from build123d import *

# Parameters (mm, degrees)
BOSS_EXTRUDE1_DEPTH       = 360
CUT_EXTRUDE1_REACH        = 4
SKETCH2_R                 = 2.25
SKETCH3_R                 = 2.25
CUT_EXTRUDE2_DEPTH        = 2
LPATTERN1_COUNT           = 5
LPATTERN1_PITCH           = 25.65625
LPATTERN2_COUNT           = 3
LPATTERN2_PITCH           = 124.1875
LPATTERN2_COPY_1_SKETCH_R = 2.25
LPATTERN2_COPY_1_DEPTH    = 2
LPATTERN2_COPY_2_SKETCH_R = 2.25
LPATTERN2_COPY_2_DEPTH    = 2
LPATTERN2_COPY_3_SKETCH_R = 2.25
LPATTERN2_COPY_3_DEPTH    = 2
LPATTERN2_COPY_4_SKETCH_R = 2.25
LPATTERN2_COPY_4_DEPTH    = 2
LPATTERN2_COPY_5_SKETCH_R = 2.25
LPATTERN2_COPY_5_DEPTH    = 2
LPATTERN2_COPY_6_SKETCH_R = 2.25
LPATTERN2_COPY_6_DEPTH    = 2
LPATTERN2_COPY_7_SKETCH_R = 2.25
LPATTERN2_COPY_7_DEPTH    = 2
LPATTERN2_COPY_8_SKETCH_R = 2.25
LPATTERN2_COPY_8_DEPTH    = 2


with BuildPart() as part:
    # Sketch1 → Boss-Extrude1 (new body)
    with BuildSketch(Plane(origin=(0, 0, 0), x_dir=(1, 0, 0), z_dir=(0, 1, 0))):
        Polygon((0, 0), (15, 0), (15, 12), (13, 12), (13, 2), (0, 2), align=None)
    extrude(amount=BOSS_EXTRUDE1_DEPTH)

    # Sketch2 → Cut-Extrude1 (cut, up to next)
    with BuildSketch(Plane.ZY.offset(-13), mode=Mode.PRIVATE) as cut_extrude1_sk1:
        with Locations((-4.5, 329.8125)):
            Circle(SKETCH2_R)
    cut_extrude1_tool1 = extrude(cut_extrude1_sk1.sketch, amount=-CUT_EXTRUDE1_REACH, mode=Mode.PRIVATE) & part.part
    add(cut_extrude1_tool1.solids().sort_by_distance((13, 329.8125, -4.5))[0], mode=Mode.SUBTRACT)
    # Sketch2 → Cut-Extrude1 (cut, up to next)
    with BuildSketch(Plane.ZY.offset(-13), mode=Mode.PRIVATE) as cut_extrude1_sk2:
        with Locations((-4.5, 304.125)):
            Circle(SKETCH2_R)
    cut_extrude1_tool2 = extrude(cut_extrude1_sk2.sketch, amount=-CUT_EXTRUDE1_REACH, mode=Mode.PRIVATE) & part.part
    add(cut_extrude1_tool2.solids().sort_by_distance((13, 304.125, -4.5))[0], mode=Mode.SUBTRACT)
    # Sketch2 → Cut-Extrude1 (cut, up to next)
    with BuildSketch(Plane.ZY.offset(-13), mode=Mode.PRIVATE) as cut_extrude1_sk3:
        with Locations((-4.5, 278.4375)):
            Circle(SKETCH2_R)
    cut_extrude1_tool3 = extrude(cut_extrude1_sk3.sketch, amount=-CUT_EXTRUDE1_REACH, mode=Mode.PRIVATE) & part.part
    add(cut_extrude1_tool3.solids().sort_by_distance((13, 278.4375, -4.5))[0], mode=Mode.SUBTRACT)
    # Sketch2 → Cut-Extrude1 (cut, up to next)
    with BuildSketch(Plane.ZY.offset(-13), mode=Mode.PRIVATE) as cut_extrude1_sk4:
        with Locations((-4.5, 252.75)):
            Circle(SKETCH2_R)
    cut_extrude1_tool4 = extrude(cut_extrude1_sk4.sketch, amount=-CUT_EXTRUDE1_REACH, mode=Mode.PRIVATE) & part.part
    add(cut_extrude1_tool4.solids().sort_by_distance((13, 252.75, -4.5))[0], mode=Mode.SUBTRACT)
    # Sketch2 → Cut-Extrude1 (cut, up to next)
    with BuildSketch(Plane.ZY.offset(-13), mode=Mode.PRIVATE) as cut_extrude1_sk5:
        with Locations((-4.5, 231.375)):
            Circle(SKETCH2_R)
    cut_extrude1_tool5 = extrude(cut_extrude1_sk5.sketch, amount=-CUT_EXTRUDE1_REACH, mode=Mode.PRIVATE) & part.part
    add(cut_extrude1_tool5.solids().sort_by_distance((13, 231.375, -4.5))[0], mode=Mode.SUBTRACT)
    # Sketch2 → Cut-Extrude1 (cut, up to next)
    with BuildSketch(Plane.ZY.offset(-13), mode=Mode.PRIVATE) as cut_extrude1_sk6:
        with Locations((-4.5, 205.6875)):
            Circle(SKETCH2_R)
    cut_extrude1_tool6 = extrude(cut_extrude1_sk6.sketch, amount=-CUT_EXTRUDE1_REACH, mode=Mode.PRIVATE) & part.part
    add(cut_extrude1_tool6.solids().sort_by_distance((13, 205.6875, -4.5))[0], mode=Mode.SUBTRACT)
    # Sketch2 → Cut-Extrude1 (cut, up to next)
    with BuildSketch(Plane.ZY.offset(-13), mode=Mode.PRIVATE) as cut_extrude1_sk7:
        with Locations((-4.5, 180)):
            Circle(SKETCH2_R)
    cut_extrude1_tool7 = extrude(cut_extrude1_sk7.sketch, amount=-CUT_EXTRUDE1_REACH, mode=Mode.PRIVATE) & part.part
    add(cut_extrude1_tool7.solids().sort_by_distance((13, 180, -4.5))[0], mode=Mode.SUBTRACT)
    # Sketch2 → Cut-Extrude1 (cut, up to next)
    with BuildSketch(Plane.ZY.offset(-13), mode=Mode.PRIVATE) as cut_extrude1_sk8:
        with Locations((-4.5, 154.3125)):
            Circle(SKETCH2_R)
    cut_extrude1_tool8 = extrude(cut_extrude1_sk8.sketch, amount=-CUT_EXTRUDE1_REACH, mode=Mode.PRIVATE) & part.part
    add(cut_extrude1_tool8.solids().sort_by_distance((13, 154.3125, -4.5))[0], mode=Mode.SUBTRACT)
    # Sketch2 → Cut-Extrude1 (cut, up to next)
    with BuildSketch(Plane.ZY.offset(-13), mode=Mode.PRIVATE) as cut_extrude1_sk9:
        with Locations((-4.5, 128.625)):
            Circle(SKETCH2_R)
    cut_extrude1_tool9 = extrude(cut_extrude1_sk9.sketch, amount=-CUT_EXTRUDE1_REACH, mode=Mode.PRIVATE) & part.part
    add(cut_extrude1_tool9.solids().sort_by_distance((13, 128.625, -4.5))[0], mode=Mode.SUBTRACT)
    # Sketch2 → Cut-Extrude1 (cut, up to next)
    with BuildSketch(Plane.ZY.offset(-13), mode=Mode.PRIVATE) as cut_extrude1_sk10:
        with Locations((-4.5, 107.25)):
            Circle(SKETCH2_R)
    cut_extrude1_tool10 = extrude(cut_extrude1_sk10.sketch, amount=-CUT_EXTRUDE1_REACH, mode=Mode.PRIVATE) & part.part
    add(cut_extrude1_tool10.solids().sort_by_distance((13, 107.25, -4.5))[0], mode=Mode.SUBTRACT)
    # Sketch2 → Cut-Extrude1 (cut, up to next)
    with BuildSketch(Plane.ZY.offset(-13), mode=Mode.PRIVATE) as cut_extrude1_sk11:
        with Locations((-4.5, 81.5625)):
            Circle(SKETCH2_R)
    cut_extrude1_tool11 = extrude(cut_extrude1_sk11.sketch, amount=-CUT_EXTRUDE1_REACH, mode=Mode.PRIVATE) & part.part
    add(cut_extrude1_tool11.solids().sort_by_distance((13, 81.5625, -4.5))[0], mode=Mode.SUBTRACT)
    # Sketch2 → Cut-Extrude1 (cut, up to next)
    with BuildSketch(Plane.ZY.offset(-13), mode=Mode.PRIVATE) as cut_extrude1_sk12:
        with Locations((-4.5, 55.875)):
            Circle(SKETCH2_R)
    cut_extrude1_tool12 = extrude(cut_extrude1_sk12.sketch, amount=-CUT_EXTRUDE1_REACH, mode=Mode.PRIVATE) & part.part
    add(cut_extrude1_tool12.solids().sort_by_distance((13, 55.875, -4.5))[0], mode=Mode.SUBTRACT)
    # Sketch2 → Cut-Extrude1 (cut, up to next)
    with BuildSketch(Plane.ZY.offset(-13), mode=Mode.PRIVATE) as cut_extrude1_sk13:
        with Locations((-4.5, 30.1875)):
            Circle(SKETCH2_R)
    cut_extrude1_tool13 = extrude(cut_extrude1_sk13.sketch, amount=-CUT_EXTRUDE1_REACH, mode=Mode.PRIVATE) & part.part
    add(cut_extrude1_tool13.solids().sort_by_distance((13, 30.1875, -4.5))[0], mode=Mode.SUBTRACT)
    # Sketch2 → Cut-Extrude1 (cut, up to next)
    with BuildSketch(Plane.ZY.offset(-13), mode=Mode.PRIVATE) as cut_extrude1_sk14:
        with Locations((-4.5, 4.5)):
            Circle(SKETCH2_R)
    cut_extrude1_tool14 = extrude(cut_extrude1_sk14.sketch, amount=-CUT_EXTRUDE1_REACH, mode=Mode.PRIVATE) & part.part
    add(cut_extrude1_tool14.solids().sort_by_distance((13, 4.5, -4.5))[0], mode=Mode.SUBTRACT)
    # Sketch2 → Cut-Extrude1 (cut, up to next)
    with BuildSketch(Plane.ZY.offset(-13), mode=Mode.PRIVATE) as cut_extrude1_sk15:
        with Locations((-4.5, 355.5)):
            Circle(SKETCH2_R)
    cut_extrude1_tool15 = extrude(cut_extrude1_sk15.sketch, amount=-CUT_EXTRUDE1_REACH, mode=Mode.PRIVATE) & part.part
    add(cut_extrude1_tool15.solids().sort_by_distance((13, 355.5, -4.5))[0], mode=Mode.SUBTRACT)

    # Sketch3 → Cut-Extrude2 (cut)
    with BuildSketch(Plane.XY):
        with Locations((7.5, 355.5)):
            Circle(SKETCH3_R)
    cut_extrude2 = extrude(amount=-CUT_EXTRUDE2_DEPTH, mode=Mode.SUBTRACT)

    # LPattern1: Cut-Extrude2 ×5
    with Locations(*[(0, -i * LPATTERN1_PITCH, 0) for i in range(1, LPATTERN1_COUNT)]):
        add(cut_extrude2, mode=Mode.SUBTRACT)

    # LPattern2: Cut-Extrude2 ×3
    with Locations(*[(0, -i * LPATTERN2_PITCH, 0) for i in range(1, LPATTERN2_COUNT)]):
        add(cut_extrude2, mode=Mode.SUBTRACT)

    # LPattern2 copy 1 sketch → LPattern2 copy 1 (cut)
    with BuildSketch(Plane(origin=(0, -149.84375, 0), x_dir=(1, 0, 0), z_dir=(0, 0, 1))):
        with Locations((7.5, 355.5)):
            Circle(LPATTERN2_COPY_1_SKETCH_R)
    extrude(amount=-LPATTERN2_COPY_1_DEPTH, mode=Mode.SUBTRACT)

    # LPattern2 copy 2 sketch → LPattern2 copy 2 (cut)
    with BuildSketch(Plane(origin=(0, -274.03125, 0), x_dir=(1, 0, 0), z_dir=(0, 0, 1))):
        with Locations((7.5, 355.5)):
            Circle(LPATTERN2_COPY_2_SKETCH_R)
    extrude(amount=-LPATTERN2_COPY_2_DEPTH, mode=Mode.SUBTRACT)

    # LPattern2 copy 3 sketch → LPattern2 copy 3 (cut)
    with BuildSketch(Plane(origin=(0, -175.5, 0), x_dir=(1, 0, 0), z_dir=(0, 0, 1))):
        with Locations((7.5, 355.5)):
            Circle(LPATTERN2_COPY_3_SKETCH_R)
    extrude(amount=-LPATTERN2_COPY_3_DEPTH, mode=Mode.SUBTRACT)

    # LPattern2 copy 4 sketch → LPattern2 copy 4 (cut)
    with BuildSketch(Plane(origin=(0, -299.6875, 0), x_dir=(1, 0, 0), z_dir=(0, 0, 1))):
        with Locations((7.5, 355.5)):
            Circle(LPATTERN2_COPY_4_SKETCH_R)
    extrude(amount=-LPATTERN2_COPY_4_DEPTH, mode=Mode.SUBTRACT)

    # LPattern2 copy 5 sketch → LPattern2 copy 5 (cut)
    with BuildSketch(Plane(origin=(0, -201.15625, 0), x_dir=(1, 0, 0), z_dir=(0, 0, 1))):
        with Locations((7.5, 355.5)):
            Circle(LPATTERN2_COPY_5_SKETCH_R)
    extrude(amount=-LPATTERN2_COPY_5_DEPTH, mode=Mode.SUBTRACT)

    # LPattern2 copy 6 sketch → LPattern2 copy 6 (cut)
    with BuildSketch(Plane(origin=(0, -325.34375, 0), x_dir=(1, 0, 0), z_dir=(0, 0, 1))):
        with Locations((7.5, 355.5)):
            Circle(LPATTERN2_COPY_6_SKETCH_R)
    extrude(amount=-LPATTERN2_COPY_6_DEPTH, mode=Mode.SUBTRACT)

    # LPattern2 copy 7 sketch → LPattern2 copy 7 (cut)
    with BuildSketch(Plane(origin=(0, -226.8125, 0), x_dir=(1, 0, 0), z_dir=(0, 0, 1))):
        with Locations((7.5, 355.5)):
            Circle(LPATTERN2_COPY_7_SKETCH_R)
    extrude(amount=-LPATTERN2_COPY_7_DEPTH, mode=Mode.SUBTRACT)

    # LPattern2 copy 8 sketch → LPattern2 copy 8 (cut)
    with BuildSketch(Plane(origin=(0, -351, 0), x_dir=(1, 0, 0), z_dir=(0, 0, 1))):
        with Locations((7.5, 355.5)):
            Circle(LPATTERN2_COPY_8_SKETCH_R)
    extrude(amount=-LPATTERN2_COPY_8_DEPTH, mode=Mode.SUBTRACT)


solid = part.part
Geometry check sheet. Reference: the model listing, model coordinates, mm. A direction names the side the tool comes from. Give positions to 0.01 mm unless a question says otherwise; leave off trailing zeros. Order: outer loops, then holes, each group sorted by start corner. A loop starts at its lowest first (then second) coordinate and runs counter-clockwise, first axis right, second up. Notation, with made-up numbers: (-23.75, -31) - (2.25, -31) arc R15 cw to (2.25, -3) - close; hole circle Ø4 at (65, -33.5). An arc over 180 degrees is marked (long way). Use one line per item in the form item = value.
1) Material ranges on probe 1 along Z at (x, y) = (14.1, 252.75); probe 2 along Z at (x, y) = (5.25, 27); probe 3 along X at (y, z) = (218, -3), recorded low to high. Write a range as from..to.
Working result:
probe_1 = -12..-6.75, -2.25..0
probe_2 = -2..0
probe_3 = 13..15
2) Sectioned sample at A-A (z = -4.5). Count the separate pieces of the cut face and the enclosed holes in it, and give its area (3 significant figures).
Working result:
separate_pieces = 16
enclosed_holes = 0
area = 585 mm^2
3) Access from +Z, -Z, +X, -X, +Y, -Y to the whole of each face (thin tool, end or side, straight path). Record for faces 1 (the face through (9.7, 360, -1.6)), 2 (the face through (13, 177, -7)).
Working result:
face_1 = +Z, -Z, +X, -X, +Y
face_2 = -Z, -X, +Y, -Y
4) Sectioned sample at B-B (y = 241). Record the boundary of the cut face in (x, z), and give its area (3 significant figures).
Working result:
outline = (0, -2) - (13, -2) - (13, -12) - (15, -12) - (15, 0) - (0, 0) - close
area = 50.0 mm^2
5) Depth check by flat-ended pin: pin 1 Ø3.5 at (x, y) = (7.5, 252.875) entering from -Z; pin 2 Ø2 at (x, y) = (7.5, 113) entering from -Z; pin 3 Ø3 at (y, z) = (105, -4.5) entering from -X. Enter the tip coordinate at first touch or a pass-through.
Working result:
pin_1 = through
pin_2 = -2
pin_3 = 13
